Source: three-view drawing plus pictorial views. Frame: mm from the lowest corner of the part. A direction names the side the tool comes from. Coordinates: 2 decimals unless noted, no trailing zeros. Write each loop counter-clockwise with the first axis right and the second up, starting at its lowest first coordinate (ties: lowest second). Pieces come first, ordered by that corner, then holes. Notation, with made-up numbers: M 27.5,86 L 55.5,86 A12 cw 55.5,93 Z; hole C 67,9 d11. An arc over 180 degrees is marked long. Write item = value, one per line. Start each with the question number.
Item 1: First-contact query: pin 1 Ø5 at (y, z) = (6.6, 8.68) entering from +X; pin 2 Ø3 at (y, z) = (7.5, 13) entering from -X; pin 3 Ø4 at (x, y) = (10.5, 20) entering from +Z; pin 4 Ø0.5 at (x, z) = (14.5, 10.5) entering from +Y. Flat tips, straight axial feed; report the tip coordinate or a pass-through.
Item 2: Section B-B on y = 9. Output: boundary loops of the cut face in (x, z).
Item 3: Section D-D on x = 7. Output: boundary loops of the cut face in (y, z).
Item 4: Section C-C on z = 4. Output: boundary loops of the cut face in (x, y) (1 decimal).
Item 5: Section A-A on z = 6.5. Output: boundary loops of the cut face in (x, y) (1 decimal).
Item 6: Ray query, L1, parallel to X at y = 11, z = 5.5; L2, parallel to Z at x = 1.75, y = 5; L3, parallel to Y at x = 14.75, z = 12.25 (1 decimal). Return the intervals inside material, ascending. Write a range as [from, to].
Item 7: Reachability of the marked faces 1 and 2 from +Z, -Z, +X, -X, +Y, -Y: full face, straight path, thin tool, end or side. Return the list, or none.
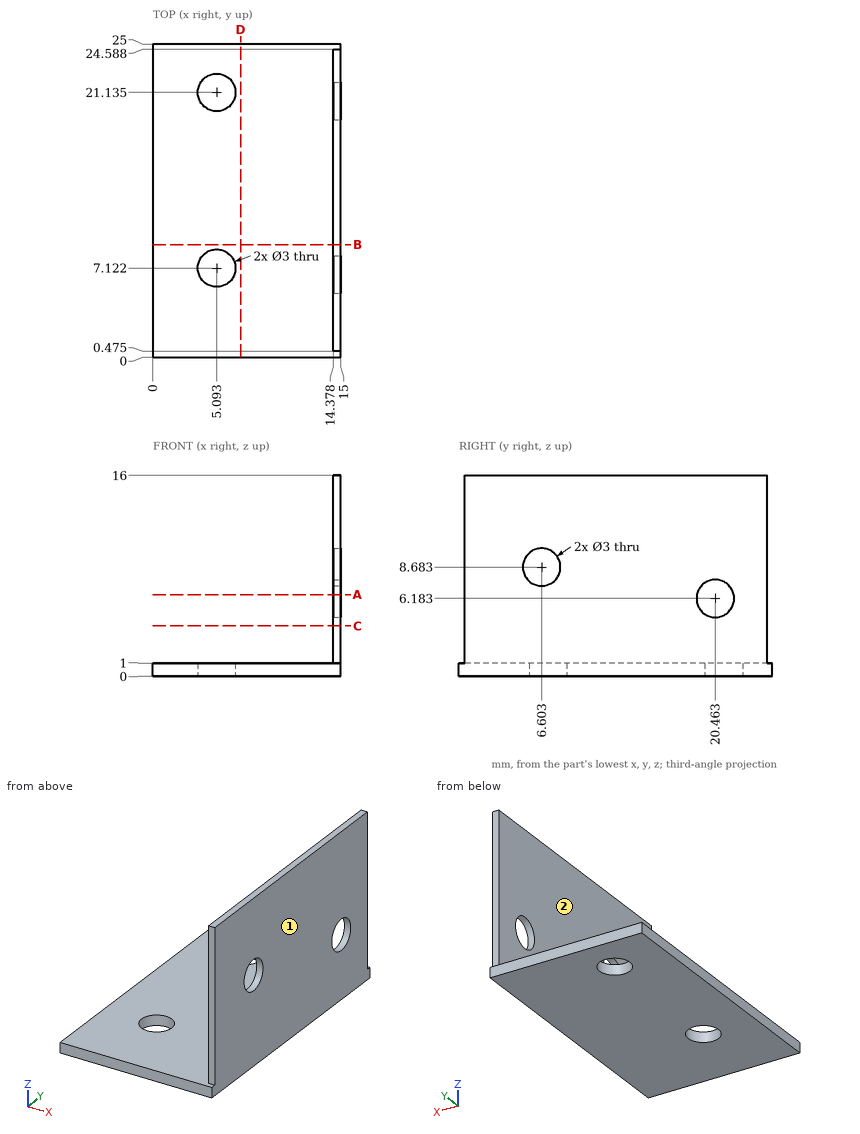
Responses:
q1.pin_1 = 15
q1.pin_2 = 14.38
q1.pin_3 = 1
q1.pin_4 = 24.59
q2.outline = M 0,0 L 15,0 L 15,16 L 14.38,16 L 14.38,1 L 0,1 Z
q3.outline = M 0,0 L 25,0 L 25,1 L 0,1 Z
q4.outline = M 14.4,0.5 L 15,0.5 L 15,24.6 L 14.4,24.6 Z
q5.outline = M 14.4,0.5 L 15,0.5 L 15,19 L 14.4,19 Z; M 14.4,21.9 L 15,21.9 L 15,24.6 L 14.4,24.6 Z
q6.L1 = [14.38, 15]
q6.L2 = [0, 1]
q6.L3 = [0.5, 24.6]
q7.face_1 = +Z, -Z, +X, +Y, -Y
q7.face_2 = +Z, -X, +Y, -Y
